from build123d import *

# Parameters (mm, degrees)
SKETCH1_R           = 3
BOSS_EXTRUDE2_DEPTH = 11.7


with BuildPart() as part:
    # Sketch1 → Boss-Extrude2 (new body)
    with BuildSketch(Plane(origin=(0, 0, 0), x_dir=(1, 0, 0), z_dir=(0, 1, 0))):
        Polygon((0, 0), (-13.980822987, 0), (-32.542943678, 31.028387767), (-17.105764768, 88.055142801), (-9.7150509, 88.055142801), (-9.7150509, 93.055142801), (-4.7150509, 93.055142801), (-4.7150509, 76.335429628), (-9.7150509, 76.335429628), (-9.7150509, 81.335429628), (-13.980822987, 81.335429628), (-22.554180854, 39.771961165), (0, 15.218862691), align=None)
        with Locations(Location((-8.736754508, 8.454923717, 0), (0, 0, 270))):
            Circle(SKETCH1_R, mode=Mode.SUBTRACT)
    extrude(amount=BOSS_EXTRUDE2_DEPTH)


solid = part.part
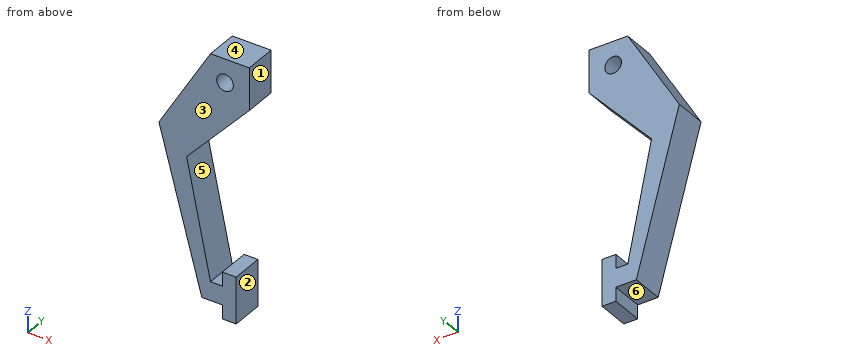
The listing builds one solid part. Answer for the finished solid, in the listing's coordinates (mm). Face numbers are marked on the shaded views. A direction names the side the tool comes from. Round coordinates to 2 decimals unless told otherwise and drop trailing zeros. Write each loop counter-clockwise with the first axis right and the second up, starting at its lowest first coordinate (ties: lowest second). Pieces come first, ordered by that corner, then holes. Notation, with made-up numbers: M 33.5,-16.5 L 73.5,-16.5 A24 ccw 73.5,20.5 Z; hole C -32.5,-9.75 d5. An arc over 180 degrees is marked long. Write each question's results on one line, items separated by ' | '. Start each with the question number.
(1) Find the intervals of material crossed by line 1 (Z direction, x = -8, y = 7.75); line 2 (Z direction, x = -10.5, y = 1.5); line 3 (X direction, y = 2.75, z = -77.5), in increasing order.
(2) For the marked faces 1 and 2, determine the directions among +Z, -Z, +X, -X, +Y, -Y from which every point of the face is accessible in a straight line to the end or side of a thin tool.
(3) Determine the mould class of the marked faces 3, 4, 5 and 6 for opening direction Z: +Z half, -Z half, draft (parallel to the pull), parting line (faces both ways), or undercut.
(4) The part is cut by section B-B, the plane z = -80.5. Write down the section's boundary in (x, y), and give its area (3 significant figures).
(5) The part is cut by section D-D, the plane z = -23. Write down the section's boundary in (x, y), and give its area (3 significant figures).
(6) Each of these flat-tipped pins is pushed along its axis until it touches: P1, Ø4, axis at x = -29, y = 7, coming from the +Z side; P2, Ø10, axis at x = -6.5, z = -68, coming from the -Y side; P3, Ø6, axis at x = -18, z = -53, coming from the +Y side; P4, Ø5.5, axis at y = 7.5, z = -89.5, coming from the -X side. Where does it stop, or does it pass through?
(7) The part is cut by section C-C, the plane y = 3.5. Write down the section's boundary in (x, z), and give its area (3 significant figures).
(8) The part is cut by section A-A, the plane x = -13. Write down the section's boundary in (y, z).
Worked answers:
1) line 1: z = -93.06 to -76.34, -23.93 to -11.36, -5.55 to 0 | line 2: z = -88.06 to -81.34, -26.65 to -10.88, -6.03 to 0 | line 3: x = -19.96 to -14.77, -9.72 to -4.72
2) face 1: +Z, -Z, +X, +Y, -Y | face 2: -Z, +X, +Y, -Y
3) face 3: draft | face 4: +Z half | face 5: undercut | face 6: -Z half
4) outline: M -19.15,0 L -14.15,0 L -14.15,11.7 L -19.15,11.7 Z; M -9.72,0 L -4.72,0 L -4.72,11.7 L -9.72,11.7 Z | area: 117 mm²
5) outline: M -27.74,0 L -7.15,0 L -7.15,11.7 L -27.74,11.7 Z | area: 241 mm²
6) P1: stops at z = -21.76 | P2: passes through | P3: stops at y = 11.7 | P4: stops at x = -17.46
7) outline: M -32.54,-31.03 L -17.11,-88.06 L -9.72,-88.06 L -9.72,-93.06 L -4.72,-93.06 L -4.72,-76.34 L -9.72,-76.34 L -9.72,-81.34 L -13.98,-81.34 L -22.55,-39.77 L 0,-15.22 L 0,0 L -13.98,0 Z; hole C -8.74,-8.45 d6 | area: 1,090 mm²
8) outline: M 0,-88.06 L 11.7,-88.06 L 11.7,-81.34 L 0,-81.34 Z; M 0,-29.37 L 11.7,-29.37 L 11.7,0 L 0,0 Z
